Work out the finished part from the listing and answer in its coordinate system (mm). Face numbers are marked on the shaded views. A direction names the side the tool comes from. Give positions to 0.01 mm unless a question says otherwise; leave off trailing zeros. Order: outer loops, then holes, each group sorted by start corner. A loop starts at its lowest first (then second) coordinate and runs counter-clockwise, first axis right, second up. Notation, with made-up numbers: M -28,79 L 8,79 A8 cw 8,91 Z; hole C -14,44.25 d2. An arc over 180 degrees is marked long. One line per item, written item: value.
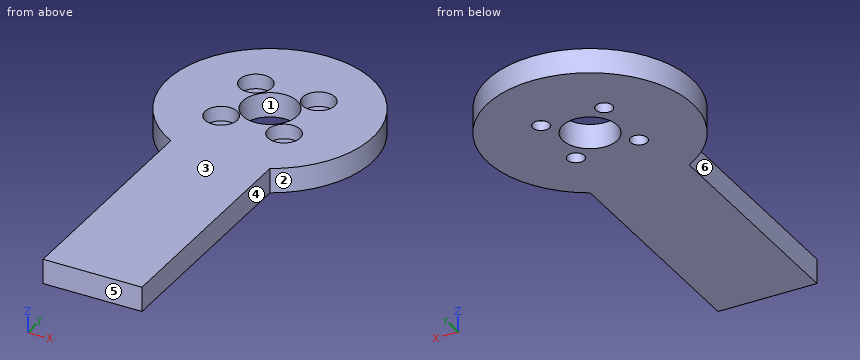
from build123d import *

# Parameters (mm, degrees)
SKETCH_1_R                  = 20.75
EXTRUDE_1_DEPTH             = 5
HOLE_WIZARD_M31_D           = 3.4
HOLE_WIZARD_M31_CBORE_D     = 6.5
HOLE_WIZARD_M31_CBORE_DEPTH = 3
SKETCH_5_R                  = 5.5
CUT_EXTRUDE_1_DEPTH         = 30.767851787
SKETCH_6_W                  = 20
SKETCH_6_H                  = 50
EXTRUDE_2_DEPTH             = 5


with BuildPart() as part:
    # Эскиз1 → Бобышка-Вытянуть1 (new body)
    with BuildSketch(Plane.XY):
        Circle(SKETCH_1_R)
    extrude(amount=EXTRUDE_1_DEPTH)

    # Цековка для винта с внутренним шестигранником M31 (through all)
    with Locations(Plane.XY.offset(5)):
        with Locations((-6.363961031, 6.363961031), (6.363961031, 6.363961031), (6.363961031, -6.363961031), (-6.363961031, -6.363961031)):
            CounterBoreHole(HOLE_WIZARD_M31_D / 2, HOLE_WIZARD_M31_CBORE_D / 2, HOLE_WIZARD_M31_CBORE_DEPTH)

    # Эскиз5 → Вырез-Вытянуть1 (cut, through all)
    with BuildSketch(Plane.XY.offset(5)):
        Circle(SKETCH_5_R)
    extrude(amount=-CUT_EXTRUDE_1_DEPTH, mode=Mode.SUBTRACT)

    # Эскиз6 → Бобышка-Вытянуть2 (add)
    with BuildSketch(Plane.XY.offset(5)):
        with Locations((0, -40)):
            Rectangle(SKETCH_6_W, SKETCH_6_H)
    extrude(amount=-EXTRUDE_2_DEPTH)


solid = part.part
(1) Section D-D, the plane y = -49 is taken. Give the vertices of the cut face in (x, z), then the cut area to 3 significant figures.
Findings:
outline: M -10,0 L 10,0 L 10,5 L -10,5 Z
area: 100 mm^2
(2) Section C-C, the plane z = 3.85 is taken. Give the vertices of the cut face in (x, y).
Findings:
outline: M -10,-65 L 10,-65 L 10,-18.18 A20.75 ccw long -10,-18.18 Z; hole C -6.36,-6.36 d6.5; hole C -6.36,6.36 d6.5; hole C 0,0 d11; hole C 6.36,-6.36 d6.5; hole C 6.36,6.36 d6.5
(3) Given P1, Ø6, axis at x = 6.36, y = -6.36, coming from the -Z side; P2, Ø2, axis at y = -53, z = 1.5, coming from the -X side; P3, Ø1, axis at x = -16, z = 3.5, coming from the +Y side; P4, Ø3, axis at x = -6, y = -7, coming from the +Z side, each flat-ended and moving along its own axis, determine where each tip first touches the part or whether it passes through.
Findings:
P1: stops at z = 0
P2: stops at x = -10
P3: stops at y = 13.8
P4: stops at z = 2
(4) Section B-B, the plane y = 2 is taken. Give the vertices of the cut face in (x, z).
Findings:
outline: M -20.65,0 L -5.12,0 L -5.12,5 L -20.65,5 Z; M 5.12,0 L 20.65,0 L 20.65,5 L 5.12,5 Z
(5) Determine the mould class of the marked faces 1, 2 and 3 for opening direction Y: pulls with the +Y half, pulls with the -Y half, needs draft (parallel to the pull), parting line crosses it, or undercut.
Findings:
face 1: undercut
face 2: parting line crosses it
face 3: needs draft
(6) Find the intervals of material crossed by probe 1 along Y at (x, z) = (0, 3); probe 2 along X at (y, z) = (-58, 3.35); probe 3 along X at (y, z) = (4, 0.6), in increasing order. Write a range as from..to.
Findings:
probe 1: y = -65..-5.5, 5.5..20.75
probe 2: x = -10..10
probe 3: x = -20.36..-3.77, 3.77..20.36
(7) Section A-A, the plane x = 0 is taken. Give the vertices of the cut face in (y, z), then the cut area to 3 significant figures.
Findings:
outline: M -65,0 L -5.5,0 L -5.5,5 L -65,5 Z; M 5.5,0 L 20.75,0 L 20.75,5 L 5.5,5 Z
area: 374 mm^2
(8) Which of the six approach directions +Z, -Z, +X, -X, +Y, -Y give full straight-line access (tool end or side, diameter ignored) to the marked faces 4, 5 and 6?
Findings:
face 4: +Z, -Z, +X, -Y
face 5: +Z, -Z, +X, -X, -Y
face 6: +Z, -Z, -X, -Y
